The listing builds one solid part. Answer for the finished solid, in the listing's coordinates (mm). A direction names the side the tool comes from. Round coordinates to 2 decimals unless told otherwise and drop trailing zeros. Write each loop counter-clockwise with the first axis right and the second up, starting at its lowest first coordinate (ties: lowest second). Pieces come first, ordered by that corner, then holes.
Item 1: Find section B-B on z = 36.5. Give the vertices of the cut face in (x, y), then the cut area to 3 significant figures.
Item 2: Find section C-C on y = 11.5. Give the vertices of the cut face in (x, z).
Item 3: Find the intervals of material crossed by probe 1 along X at (y, z) = (7.5, 51); probe 2 along Y at (x, z) = (17, 60); probe 3 along Z at (x, y) = (62, -15), in increasing order.
Item 4: A tool of negligible diameter and unlimited length cuts with its end or side. For faces 4 (the face through (-1, -45, 51)), 5 (the face through (-105, 0, 52)), 6 (the face through (100, -1, 49)), from which of +Z, -Z, +X, -X, +Y, -Y can it reach the whole face along a straight path? Write none if from no direction.
Item 5: Each of these flat-tipped pins is pushed along its axis until it touches: pin 1 (1 mm diameter, centred on y = 21.5, z = 86.5, fed in from -X); pin 2 (2 mm diameter, centred on x = -24, z = 83, fed in from -Y); pin 3 (3 mm diameter, centred on x = -32, y = 38, fed in from +Z). Where does it stop, or does it pass through?
Item 6: Find section D-D on y = 33. Give the vertices of the cut face in (x, z).
Item 7: For a pull along X with two mould halves and no side action, classify faces 1 (the face through (-100, -1, 38)), 2 (the face through (-1, 1, 10)), 3 (the face through (97, 0, 100)) as +X half, -X half, draft (parallel to the pull), parting line (faces both ways), or undercut.
```python
from build123d import *

# Parameters (mm, degrees)
SKETCH_2_W          = 200
SKETCH_2_H          = 100
EXTRUDE_1_DEPTH     = 100
SKETCH_3_W          = 190
SKETCH_3_H          = 90
CUT_EXTRUDE_1_DEPTH = 90
FILLET_1_R          = 25
SKETCH_4_R          = 2
EXTRUDE_2_DEPTH     = 10


with BuildPart() as part:
    # 草图2 → 凸台-拉伸1 (new body)
    with BuildSketch(Plane.XY):
        Rectangle(SKETCH_2_W, SKETCH_2_H)
    extrude(amount=EXTRUDE_1_DEPTH)

    # 草图3 → 切除-拉伸1 (cut)
    with BuildSketch(Plane.XY.offset(100)):
        Rectangle(SKETCH_3_W, SKETCH_3_H)
    extrude(amount=-CUT_EXTRUDE_1_DEPTH, mode=Mode.SUBTRACT)

    # 圆角1
    # the kernel refuses this fillet: 25 mm, written as the material it takes off along each edge
    with BuildSketch(Plane(origin=(162.5, 50, 0), x_dir=(0, -1, 0), z_dir=(-1, 0, 0)), Plane(origin=(-162.5, -50, 100), x_dir=(0, 0, -1), z_dir=(1, 0, 0))) as fillet_1_piece_1:
        with BuildLine():
            CenterArc((FILLET_1_R, FILLET_1_R), FILLET_1_R, 180, 90)
            Line((0, FILLET_1_R), (0, 0))
            Line((0, 0), (FILLET_1_R, 0))
        make_face()
    extrude(amount=325, mode=Mode.SUBTRACT)
    with BuildSketch(Plane(origin=(-162.5, -50, 0), x_dir=(0, 0, 1), z_dir=(1, 0, 0)), Plane(origin=(162.5, 50, 100), x_dir=(0, -1, 0), z_dir=(-1, 0, 0))) as fillet_1_piece_2:
        with BuildLine():
            CenterArc((FILLET_1_R, -FILLET_1_R), FILLET_1_R, 90, 90)
            Line((0, -FILLET_1_R), (0, 0))
            Line((0, 0), (FILLET_1_R, 0))
        make_face()
    extrude(amount=325, mode=Mode.SUBTRACT)

    # 草图4 → 凸台-拉伸2 (add)
    with BuildSketch(Plane.ZY.offset(100)):
        with Locations(Location((50, 0, 0), (0, 0, 180))):
            Circle(SKETCH_4_R)
    extrude(amount=EXTRUDE_2_DEPTH)


solid = part.part
```
Check values:
1. outline: (-100, -50) - (100, -50) - (100, 50) - (-100, 50) - close; hole (-95, -45) - (95, -45) - (95, 45) - (-95, 45) - close
1. area: 2,900 mm2
2. outline: (-100, 0) - (100, 0) - (100, 100) - (95, 100) - (95, 10) - (-95, 10) - (-95, 100) - (-100, 100) - close
3. probe 1: x = -100 to -95, 95 to 100
3. probe 2: y = -50 to -45, 45 to 50
3. probe 3: z = 0 to 10
4. face 4: +Z
4. face 5: -X
4. face 6: +Z, -Z, +X, +Y, -Y
5. pin 1: stops at x = -100
5. pin 2: stops at y = -49
5. pin 3: stops at z = 10
6. outline: (-100, 1.31) - (100, 1.31) - (100, 98.69) - (95, 98.69) - (95, 10) - (-95, 10) - (-95, 98.69) - (-100, 98.69) - close
7. face 1: -X half
7. face 2: undercut
7. face 3: draft
